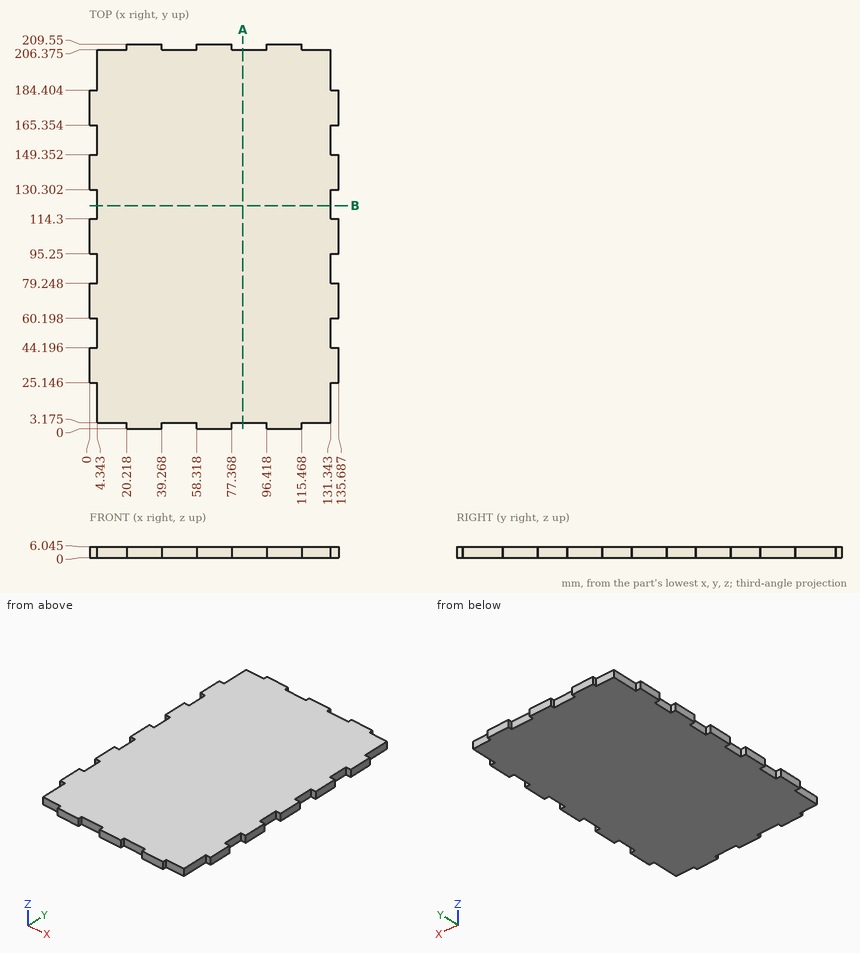
Answer from the drawing. Dimensions are ordinates in mm from the lowest x, y and z of the part. Give positions to 0.01 mm unless a question says otherwise; leave off trailing zeros. Write each loop counter-clockwise with the first axis right and the second up, starting at its lowest first coordinate (ties: lowest second). Pieces come first, ordered by that corner, then holes.
1) Section A-A (x = 83.5) is taken. Write down the section's boundary in (y, z) (1 decimal).
2) Section B-B (y = 121.5) is taken. Write down the section's boundary in (x, z) (1 decimal).
3) Find the intervals of material crossed by L1, parallel to X at y = 93.5, z = 1.5; L2, parallel to Y at x = 11, z = 4.25 (1 decimal), in increasing order.
4) Given P1, Ø3.5, axis at x = 1.5, z = 4.5, coming from the -Y side; P2, Ø1.8, axis at x = 122.5, z = 4, coming from the +Y side (3 decimals); P3, Ø1.8, axis at x = 123.5, z = 1.5, coming from the -Y side (3 decimals), each flat-ended and moving along its own axis, determine where each tip first touches the part or whether it passes through.
Response:
1. outline: (3.2, 0) - (206.4, 0) - (206.4, 6) - (3.2, 6) - close
2. outline: (4.3, 0) - (131.3, 0) - (131.3, 6) - (4.3, 6) - close
3. L1: x = 4.34 to 131.34
3. L2: y = 3.2 to 206.4
4. P1: stops at y = 25.15
4. P2: stops at y = 206.375
4. P3: stops at y = 3.175
